The listing builds one solid part. Answer for the finished solid, in the listing's coordinates (mm). Face numbers are marked on the shaded views. A direction names the side the tool comes from. Give positions to 0.01 mm unless a question says otherwise; leave off trailing zeros. Write each loop counter-clockwise with the first axis right and the second up, starting at its lowest first coordinate (ties: lowest second). Pieces come first, ordered by that corner, then holes. Notation, with made-up numbers: M 59,37 L 73,37 A26 cw 73,64 Z; hole C 0.25,-13.5 d5. An arc over 180 degrees is marked long. Answer as a JSON object with one key per item and string values.
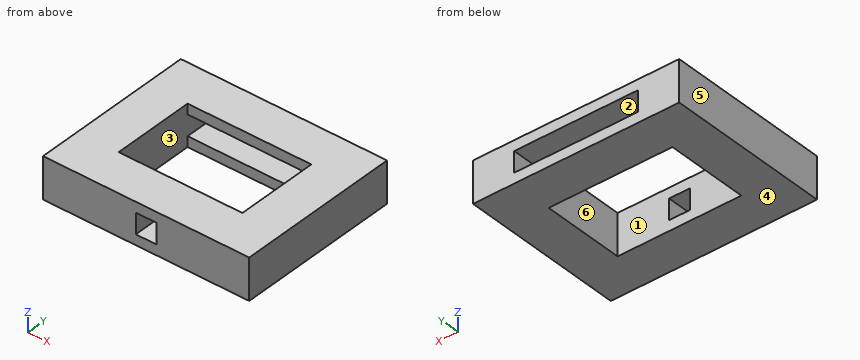
```python
from build123d import *

# Parameters (mm, degrees)
F0_W     = 50
F0_H     = 40
F0_W_2   = 30
F0_H_2   = 20
F1_DEPTH = 10
F2_W     = 30
F2_H     = 5
F3_DEPTH = 25
F4_W     = 5
F4_H     = 5
F5_DEPTH = 10


with BuildPart() as f1:
    # F0 (on Top) → F1 (new body)
    with BuildSketch(Plane.XY):
        Rectangle(F0_W, F0_H)
        Rectangle(F0_W_2, F0_H_2, mode=Mode.SUBTRACT)
    extrude(amount=F1_DEPTH)

    # F2 (on face) → F3 (cut)
    with BuildSketch(Plane(origin=(0, 20, 0), x_dir=(-1, 0, 0), z_dir=(0, 1, 0))):
        with Locations((0, 5)):
            Rectangle(F2_W, F2_H)
    extrude(amount=-F3_DEPTH, mode=Mode.SUBTRACT)

    # F4 (on face) → F5 (cut, through all)
    with BuildSketch(Plane(origin=(0, -10, 0), x_dir=(-1, 0, 0), z_dir=(0, 1, 0))):
        with Locations((0, 5)):
            Rectangle(F4_W, F4_H)
    extrude(amount=-F5_DEPTH, mode=Mode.SUBTRACT)


solid = f1.part
```
1. The mould has two halves that part along X. Classify the marked faces 4, 5 and 6: released by +X, released by -X, zero draft, split by the parting line, or undercut.
Verdict:
{"face 4": "zero draft", "face 5": "released by -X", "face 6": "undercut"}
2. For the marked faces 1, 2 and 3, determine the directions among +Z, -Z, +X, -X, +Y, -Y from which every point of the face is accessible in a straight line to the end or side of a thin tool.
Verdict:
{"face 1": "+Z, -Z", "face 2": "+Y", "face 3": "none"}
3. A cutting plane is placed at A-A, the plane x = 8. Give the vertices of the cut face in (y, z), plus the area to 3 significant figures.
Verdict:
{"outline": "M -20,0 L -10,0 L -10,10 L -20,10 Z; M 10,0 L 20,0 L 20,2.5 L 10,2.5 Z; M 10,7.5 L 20,7.5 L 20,10 L 10,10 Z", "area": "150 mm2"}
4. A cutting plane is placed at C-C, the plane z = 5.5. Give the vertices of the cut face in (x, y).
Verdict:
{"outline": "M -25,-20 L -2.5,-20 L -2.5,-10 L -15,-10 L -15,20 L -25,20 Z; M 2.5,-20 L 25,-20 L 25,20 L 15,20 L 15,-10 L 2.5,-10 Z"}
5. A cutting plane is placed at D-D, the plane y = 4. Give the vertices of the cut face in (x, z), plus the area to 3 significant figures.
Verdict:
{"outline": "M -25,0 L -15,0 L -15,10 L -25,10 Z; M 15,0 L 25,0 L 25,10 L 15,10 Z", "area": "200 mm2"}
6. A cutting plane is placed at B-B, the plane y = 15. Give the vertices of the cut face in (x, z), plus the area to 3 significant figures.
Verdict:
{"outline": "M -25,0 L 25,0 L 25,10 L -25,10 Z; hole M -15,2.5 L 15,2.5 L 15,7.5 L -15,7.5 Z", "area": "350 mm2"}
7. Consider line 1 along Z through (x, y) = (6, 17); line 2 along X through (y, z) = (-4, 8); line 3 along Y through (x, z) = (6, 0.75). Determine where each line is inside the solid, lowest interval first.
Verdict:
{"line 1": "z = 0 to 2.5, 7.5 to 10", "line 2": "x = -25 to -15, 15 to 25", "line 3": "y = -20 to -10, 10 to 20"}
